Part model, mm, in its own coordinate system. A direction names the side the tool comes from. Coordinates: 2 decimals unless noted, no trailing zeros. Order: outer loops, then holes, each group sorted by start corner. A loop starts at its lowest first (then second) coordinate and runs counter-clockwise, first axis right, second up. Notation, with made-up numbers: (-3.5, 43) - (41.5, 43) arc R19 ccw to (41.5, 77) - close; hole circle Ø7 at (44, -30). An arc over 180 degrees is marked (long way). Use a Markdown table: item, result. Add a question column.
1) Tool access for faces 1 (the face through (132.15, -7.6, 171.99)), 2 (the face through (-119.307, -7.395, -240.14)), 3 (the face through (175, -7, -16)): list every direction of +Z, -Z, +X, -X, +Y, -Y with a clear straight run to the whole face (end or side of a thin tool).
2) Wall check: L1, parallel to Z at x = -14, y = -6.5; L2, parallel to Z at x = 150, y = -5; L3, parallel to X at y = -7.75, z = 68.5. Give the ranges that are in metal, low to high. Write a range as [from, to].
3) Saw through at C-C on x = 18. List the corners of the cut face in (y, z).
4) Saw through at B-B on z = -48. List the corners of the cut face in (x, y).
5) Drop a flat-ended pin along its axis: P1, Ø7.5, axis at x = 55.5, y = -9.5, coming from the -Z side. Give the stop position or say it passes through.
6) Two-plate mould, pull along X, no slides. Class faces 4 (the face through (150, -7, -250)), 5 (the face through (-140.763, -7.395, 221.17)), 6 (the face through (167.871, -7.395, 242.482)): +X half, -X half, draft (parallel to the pull), parting line (faces both ways), or undercut.
7) Saw through at A-A on y = -4.5. List the corners of the cut face in (x, z).
```python
from build123d import *

# Parameters (mm, degrees)
F0_R     = 10
F1_DEPTH = 15
F3_DEPTH = 15.001


with BuildPart() as f1:
    # F0 (on Front) → F1 (new body)
    with BuildSketch(Plane.XZ):
        with BuildLine():
            Line((150, 250), (-150, 250))
            ThreePointArc((-150, 250), (-167.67767, 242.67767), (-175, 225))
            Line((-175, 225), (-175, -250))
            Line((-175, -250), (-125, -250))
            Line((-125, -250), (-113.452995, -230))
            Line((-113.452995, -230), (0, -230))
            Line((0, -230), (113.452995, -230))
            Line((113.452995, -230), (125, -250))
            Line((125, -250), (175, -250))
            Line((175, -250), (175, 225))
            ThreePointArc((175, 225), (167.67767, 242.67767), (150, 250))
        make_face()
        with Locations((-150, 225)):
            Circle(F0_R, mode=Mode.SUBTRACT)
        with BuildLine():
            Line((105, 210), (-105, 210))
            ThreePointArc((-105, 210), (-115, 220), (-105, 230))
            Line((-105, 230), (105, 230))
            ThreePointArc((105, 230), (115, 220), (105, 210))
        make_face(mode=Mode.SUBTRACT)
        with Locations((150, 225)):
            Circle(F0_R, mode=Mode.SUBTRACT)
    extrude(amount=F1_DEPTH)

    # F2 (on face) → F3 (cut, through all)
    with BuildSketch(Plane.XZ.offset(15)):
        with BuildLine():
            ThreePointArc((135, 165), (132.071068, 172.071068), (125, 175))
            Line((125, 175), (-125, 175))
            ThreePointArc((-125, 175), (-132.071068, 172.071068), (-135, 165))
            Line((-135, 165), (-135, -176.264953))
            ThreePointArc((-135, -176.264953), (-132.071068, -183.336021), (-125, -186.264953))
            Line((-125, -186.264953), (125, -186.264953))
            ThreePointArc((125, -186.264953), (132.071068, -183.336021), (135, -176.264953))
            Line((135, -176.264953), (135, 165))
        make_face()
    extrude(amount=-F3_DEPTH, mode=Mode.SUBTRACT)


solid = f1.part
```
Results are:
| question | item | result |
|---|---|---|
| 1 | face 1 | +Y, -Y |
| 1 | face 2 | -Z, +Y, -Y |
| 1 | face 3 | +Z, -Z, +X, +Y, -Y |
| 2 | L1 | [-230, -186.26], [175, 210], [230, 250] |
| 2 | L2 | [-250, 215], [235, 250] |
| 2 | L3 | [-175, -135], [135, 175] |
| 3 | outline | (-15, -230) - (0, -230) - (0, -186.26) - (-15, -186.26) - close; (-15, 175) - (0, 175) - (0, 210) - (-15, 210) - close; (-15, 230) - (0, 230) - (0, 250) - (-15, 250) - close |
| 4 | outline | (-175, -15) - (-135, -15) - (-135, 0) - (-175, 0) - close; (135, -15) - (175, -15) - (175, 0) - (135, 0) - close |
| 5 | P1 | z = -230 |
| 6 | face 4 | draft |
| 6 | face 5 | undercut |
| 6 | face 6 | +X half |
| 7 | outline | (-175, -250) - (-125, -250) - (-113.45, -230) - (113.45, -230) - (125, -250) - (175, -250) - (175, 225) arc R25 ccw to (150, 250) - (-150, 250) arc R25 ccw to (-175, 225) - close; hole circle Ø20 at (-150, 225); hole (-135, -176.26) arc R10 ccw to (-125, -186.26) - (125, -186.26) arc R10 ccw to (135, -176.26) - (135, 165) arc R10 ccw to (125, 175) - (-125, 175) arc R10 ccw to (-135, 165) - close; hole (-105, 210) - (105, 210) arc R10 ccw to (105, 230) - (-105, 230) arc R10 ccw to start; hole circle Ø20 at (150, 225) |
